Autodesk Inventor part; units mm, degrees
ref_plane "YZ Plane" through (0, 0, 0) normal (1, 0, 0) x (0, 1, 0)
ref_plane "XZ Plane" through (0, 0, 0) normal (0, 1, 0) x (-1, 0, 0)
ref_plane "XY Plane" through (0, 0, 0) normal (0, 0, 1) x (1, 0, 0)
sketch "Sketch1" plane through (0, 0, 0) normal (0, 1, 0) x (-1, 0, 0)
  circle A0 centre (0, 0) radius 1.4732
  circle A1 centre (0, -80.9498) radius 1.4732
  circle A2 centre (0, 0) radius 5.0165
  circle A3 centre (0, -80.9498) radius 5.0165
  line L0 (0, 5.0165) -> (4.033, 5.0165)
  line L1 (4.033, -85.9663) -> (0, -85.9663)
  line L2 (10.033, -79.9663) -> (10.033, -0.9835)
  line L3 (0, -5.0165) -> (-0.9835, -5.0165)
  line L4 (5.0165, -11.0165) -> (5.0165, -69.9333)
  line L5 (-0.9835, -75.9333) -> (0, -75.9333)
  arc A4 (10.033, -0.9835) -> (4.033, 5.0165) centre (4.033, -0.9835) ccw
  arc A5 (4.033, -85.9663) -> (10.033, -79.9663) centre (4.033, -79.9663) ccw
  arc A6 (5.0165, -11.0165) -> (-0.9835, -5.0165) centre (-0.9835, -11.0165) ccw
  arc A7 (-0.9835, -75.9333) -> (5.0165, -69.9333) centre (-0.9835, -69.9333) ccw
  point P0 (10.033, 5.0165)
  dimension "d0" = 2.9464
  dimension "d2" = 2.9464
  dimension "d3" = 10.033
  dimension "d4" = 10.033
  dimension "d7" = 80.9498
  dimension "d8" = 10.033
  dimension "d9" = 6
  dimension "d10" = 6
  dimension "d11" = 6
  dimension "d12" = 6
extrude "Extrusion1" add sketch "Sketch1" along normal blind 3.5
sketch "Sketch2" plane through (-10.033, 0, -79.9663) normal (-1, 0, 0) x (0, 0, 1)
  line L0 (0, 0) -> (0, 3.5)
  line L1 (0, 0) -> (7.62, 0)
  line L2 (0, 0) -> (78.9828, 0)
  line L3 (7.62, 0) -> (7.62, -22.225)
  line L4 (7.62, 0) -> (71.374, 0)
  line L5 (68.9498, 0) -> (10.033, 0)
  line L6 (71.374, 0) -> (71.374, -22.225)
  line L7 (68.199, -25.4) -> (10.795, -25.4)
  line L8 (7.62, 0) -> (19.2419, 0) construction
  line L9 (71.374, 0) -> (44.6419, 0) construction
  line L10 (61.849, -6.35) -> (17.145, -6.35)
  line L11 (17.145, -19.05) -> (61.849, -19.05)
  line L12 (65.024, -15.875) -> (65.024, -9.525)
  line L13 (13.97, -9.525) -> (13.97, -15.875)
  arc A0 (17.145, -6.35) -> (13.97, -9.525) centre (17.145, -9.525) ccw
  arc A1 (65.024, -9.525) -> (61.849, -6.35) centre (61.849, -9.525) ccw
  arc A2 (61.849, -19.05) -> (65.024, -15.875) centre (61.849, -15.875) ccw
  arc A3 (13.97, -15.875) -> (17.145, -19.05) centre (17.145, -15.875) ccw
  arc A4 (7.62, -22.225) -> (10.795, -25.4) centre (10.795, -22.225) ccw
  arc A5 (68.199, -25.4) -> (71.374, -22.225) centre (68.199, -22.225) ccw
  point P0 (79.9663, 0)
  point P1 (7.62, -25.4)
  point P2 (13.97, -6.35)
  point P3 (71.374, 0)
  dimension "d15" = 7.62
  dimension "d16" = 25.4
  dimension "d17" = 63.754
  dimension "d19" = 6.35
  dimension "d22" = 3.175
  dimension "d23" = 3.175
  dimension "d24" = 3.175
  dimension "d25" = 3.175
  dimension "d26" = 3.175
  dimension "d27" = 3.175
  dimension "d33" = 44.704
  dimension "d34" = 44.704
extrude "Extrusion2" add sketch "Sketch2" along normal blind 3.5
sketch "Sketch4" plane through (-10.033, 0, -8.5923) normal (0, 1, 0) x (1, 0, 0)
  line L0 (0, 63.754) -> (-3.5, 63.754)
  line L1 (0, 63.754) -> (-3.5, 63.754)
  line L2 (0, 0) -> (-3.5, 0)
  line L3 (-3.5, 63.754) -> (-3.5, 0)
  line L4 (-3.5, 0) -> (0, 0)
  line L5 (0, 0) -> (0, 63.754)
  point P0 (10.033, -8.5923)
extrude "Extrusion3" add sketch "Sketch4" along normal blind 3.5
fillet "Fillet1" radius 3.175 1 edges at (-13.533, 3.5, -40.4693)
properties part number "sidemount3"
Check sheet for the modelled part. Datum: model origin and axes. Units: mm. A direction names the side the tool comes from. Round coordinates to 2 decimals unless told otherwise and drop trailing zeros. Order: outer loops, then holes, each group sorted by start corner. A loop starts at its lowest first (then second) coordinate and runs counter-clockwise, first axis right, second up. Notation, with made-up numbers: (20.5, 87.5) -> (57.5, 87.5) arc R22 cw to (57.5, 94.5) -> close; hole circle Ø10 at (0.25, -25.5). An arc over 180 degrees is marked (long way). One line per item, written item: value. Start each with the question number.
Q1. Thickness scan on line 1 (X direction, y = -23, z = -18.5); line 2 (Y direction, x = -5.5, z = -2); line 3 (Z direction, x = -12, y = -4.75). Record the ranges inside material, lowest first.
Q2. Cross-section at B-B (y = -7.75). Record the boundary of the cut face in (x, z).
Q3. Gauge pin test, flat ends, axial feed: pin 1 Ø4 at (y, z) = (-6.5, -21) entering from +X; pin 2 Ø3 at (y, z) = (2, -76) entering from -X; pin 3 Ø4 at (x, y) = (-12.5, -12.5) entering from -Z. Record the tip position at first contact, or that the pin passes through.
Q4. Mould release check, pull along Y, two halves, no side actions. Record for faces 1 (the face through (-11.758, -7.255, -15.897)), 2 (the face through (-11.76, -24.45, -9.5)), 3 (the face through (-12.578, 2.595, -40.023)), 4 (the face through (-12, -10, -8.592)): pulls with the +Y half, pulls with the -Y half, needs draft (parallel to the pull), parting line crosses it, or undercut.
Q5. Set-up check for faces 5 (the face through (-11.758, -18.145, -65.042)), 6 (the face through (-10.033, 2, -5)), 7 (the face through (-6, 0, -40)), 8 (the face through (-3.306, 1.726, -74.129)): record each of +Z, -Z, +X, -X, +Y, -Y from which the full face is reachable in a straight line by a thin tool's end or side.
Completed:
1. line 1: x = -13.53 to -10.03
1. line 2: y = 0 to 3.5
1. line 3: z = -72.35 to -8.59
2. outline: (-13.53, -72.35) -> (-10.03, -72.35) -> (-10.03, -65.45) -> (-13.53, -65.45) -> close; (-13.53, -15.48) -> (-10.03, -15.48) -> (-10.03, -8.59) -> (-13.53, -8.59) -> close
3. pin 1: stops at x = -10.03
3. pin 2: stops at x = -10.03
3. pin 3: stops at z = -72.35
4. face 1: undercut
4. face 2: pulls with the -Y half
4. face 3: pulls with the +Y half
4. face 4: needs draft
5. face 5: +X, -X
5. face 6: +Z, -X, +Y, -Y
5. face 7: +Z, -Z, +X, -Y
5. face 8: +X, +Y, -Y
